```python
from build123d import *

# Parameters (mm, degrees)
F0_W     = 15
F0_H     = 5
F0_W_2   = 5
F0_H_2   = 35
F1_DEPTH = 34
F2_W     = 5
F2_H     = 10
F3_DEPTH = 34
F4_W     = 16.2579220422
F4_H     = 42.7319623083
F5_DEPTH = 26


with BuildPart() as f1:
    # F0 (on Front) → F1 (new body, symmetric)
    with BuildSketch(Plane.XZ):
        Polygon((-22.3241779208, 0), (30.6758220792, 0), (30.6758220792, 5), (-27.3241779208, 5), (-27.3241779208, 0), align=None)
        with Locations((-34.8241779208, 2.5)):
            Rectangle(F0_W, F0_H)
        with BuildLine():
            Line((-27.3241779208, -35), (-27.3241779208, 0))
            Line((-27.3241779208, 0), (-42.3241779208, 0))
            add(Edge.make_bspline(
                [(-42.3241779208, 0), (-32.1847312152, -6.594858598), (-28.7573114038, -19.590485841), (-27.3241779208, -35)],
                knots=[0, 0, 0, 0, 38.0788655293, 38.0788655293, 38.0788655293, 38.0788655293], degree=3))
        make_face()
        with Locations((-24.8241779208, -17.5)):
            Rectangle(F0_W_2, F0_H_2)
        Polygon((37.6758220792, -35), (-22.3241779208, -35), (-27.3241779208, -35), (-27.3241779208, -40), (37.6758220792, -40), align=None)
    extrude(amount=F1_DEPTH, both=True)

    # F2 (on Front) → F3 (join, symmetric)
    with BuildSketch(Plane.XZ):
        with Locations((-44.8241779208, 5)):
            Rectangle(F2_W, F2_H)
        with BuildLine():
            Line((-47.3241779208, 10), (-42.3241779208, 10))
            add(Edge.make_bspline(
                [(-47.3241779208, 10), (-47.1237004262, 11.8566387437), (-45.3455906765, 15.4385356924), (-41.5967992059, 13.7724758931), (-42.9261420784, 11.4005931192), (-42.3241779208, 10)],
                knots=[0, 0, 0, 0, 0.3979300769, 0.66673524, 1, 1, 1, 1], degree=3))
        make_face()
    extrude(amount=F3_DEPTH, both=True)

    # F4 (on Front) → F5 (cut, symmetric)
    with BuildSketch(Plane.XZ):
        with Locations((-43.4531389419, 0.3948621452)):
            Rectangle(F4_W, F4_H)
    extrude(amount=F5_DEPTH, both=True, mode=Mode.SUBTRACT)


solid = f1.part
```
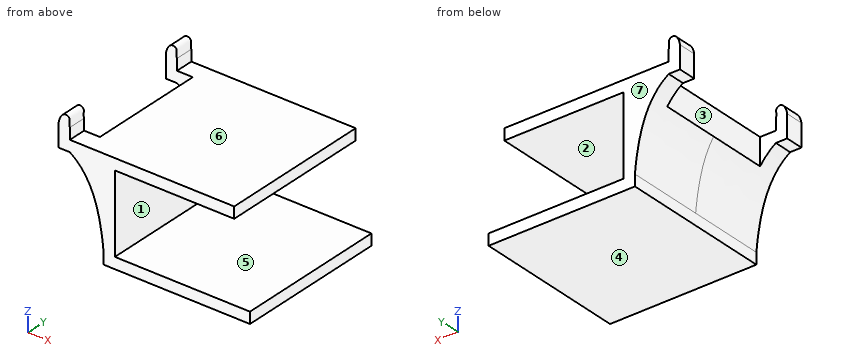
CAD build for the part. Positions are in the model's coordinates, mm. Face numbers are marked on the shaded views. A direction names the side the tool comes from. Coordinates: 2 decimals unless noted, no trailing zeros. Write each loop counter-clockwise with the first axis right and the second up, starting at its lowest first coordinate (ties: lowest second). Pieces come first, ordered by that corner, then holes.
(1) Cut at C-C, the plane z = -36. List the corners of the cut face in (x, y), and give its area (3 significant figures).
(2) Cut at A-A, the plane z = 9. List the corners of the cut face in (x, y).
(3) Drill centre lines: probe 1 along Z at (x, y) = (1, 6.5); probe 2 along X at (y, z) = (2, -4); probe 3 along Z at (x, y) = (-22.5, -2). Where is each one in solid material? Low to high.
(4) Two-plate mould, pull along Z, no slides. Class the marked faces 1, 2, 3 and 4: +Z half, -Z half, draft (parallel to the pull), parting line (faces both ways), or undercut.
(5) Cut at B-B, the plane x = 10.5. List the corners of the cut face in (y, z), and give its area (3 significant figures).
(6) 3-axis set-ups, long thin cutter, end or side, ignore diameter. For the marked faces 5, 6 and 7: which of +Z, -Z, +X, -X, +Y, -Y reach the whole face in a straight line?
(7) Flat gauge pins, fed straight in: pin 1 (3 mm diameter, centred on y = 3.5, z = -29.5, fed in from -X); pin 2 (1.5 mm diameter, centred on y = 31, z = 7.5, fed in from +X); pin 3 (1.5 mm diameter, centred on y = -1.5, z = -37, fed in from -X); pin 4 (1 mm diameter, centred on x = 27.5, z = -1, fed in from +Y). Where does each tip first touch, or does it go through?
Geometry says:
1. outline: (-27.32, -34) - (37.68, -34) - (37.68, 34) - (-27.32, 34) - close
1. area: 4,420 mm2
2. outline: (-47.32, -34) - (-42.32, -34) - (-42.32, -26) - (-47.32, -26) - close; (-47.32, 26) - (-42.32, 26) - (-42.32, 34) - (-47.32, 34) - close
3. probe 1: z = -40 to -35, 0 to 5
3. probe 2: x = -35.32 to -22.32
3. probe 3: z = -40 to 5
4. face 1: undercut
4. face 2: undercut
4. face 3: draft
4. face 4: -Z half
5. outline: (-34, -40) - (34, -40) - (34, -35) - (-34, -35) - close; (-34, 0) - (34, 0) - (34, 5) - (-34, 5) - close
5. area: 680 mm2
6. face 5: +X, +Y, -Y
6. face 6: +Z, +X, +Y, -Y
6. face 7: +Z, -Z, +X, -X, +Y
7. pin 1: stops at x = -28.16
7. pin 2: stops at x = -42.32
7. pin 3: stops at x = -27.32
7. pin 4: passes through
